Geometry check sheet. Reference: the model listing, model coordinates, mm. Face numbers are marked on the shaded views. Round coordinates to 2 decimals unless told otherwise and drop trailing zeros. Order: outer loops, then holes, each group sorted by start corner. A loop starts at its lowest first (then second) coordinate and runs counter-clockwise, first axis right, second up.
(1) Thickness scan on L1, parallel to Y at x = 0.95, z = 0; L2, parallel to Z at x = 2.2, y = -5.25. Record the ranges inside material, lowest first.
(2) Cross-section at D-D on y = -8. Enter the section's corners in (x, z).
(3) Cross-section at C-C on x = 1.4. Enter the section's corners in (y, z).
(4) Cross-section at A-A on y = 0. Enter the section's corners in (x, z).
(5) Cross-section at B-B on z = -4. Enter the section's corners in (x, y), and give its area (3 significant figures).
(6) Gauge pin test, flat ends, axial feed: P1, Ø10, axis at y = -7, z = -0.5, coming from the -X side; P2, Ø1.5, axis at x = 0.5, y = -1, coming from the +Z side. Record the tip position at first contact, or that the pin passes through.
(7) Draft check along X on the marked faces 1 and 2. Enter one of: pulls with the +X half, pulls with the -X half, needs draft (parallel to the pull), parting line crosses it, or undercut.
Autodesk Inventor part; units mm, degrees
ref_plane "Work Plane1" through (0, 0, 0) normal (0, -1, 0) x (1, 0, 0)
ref_plane "YZ Plane" through (0, 0, 0) normal (1, 0, 0) x (0, 1, 0)
ref_plane "XZ Plane" through (0, 0, 0) normal (0, 1, 0) x (-1, 0, 0)
sketch "草图1" plane through (0, 0, 0) normal (1, 0, 0) x (0, 1, 0)
  circle A0 centre (0, 0) radius 9.2
  circle A1 centre (0, 0) radius 6.1
  dimension "d0" = 12.2
  dimension "d1" = 18.4
extrude "轴承体" add sketch "草图1" along normal blind 3.1
sketch "草图2" plane through (0, 0, 0) normal (0, 0, 1) x (1, 0, 0)
  line L0 (0, -6.1) -> (0, 6.1)
  line L1 (3.1, 9.2) -> (3.1, -9.2)
  line L2 (-1.2, 0) -> (7.2, 0)
  line L3 (0, -0.62) -> (3.1, 0.3873)
  line L4 (0, 0.62) -> (3.1, 1.6273)
  dimension "d4" = 0.62
  dimension "d5" = 0.62
  dimension "d6" = 72
extrude "切口" cut sketch "草图2" along normal up to next contours L0 L2 L3 | L0 L4 L1 L3 L2
ref_plane "Work Plane1" through (0, 0, 0) normal (0, -1, 0) x (1, 0, 0)
equation "\"d0\" = SD1"
equation "\"d1\" = SD2"
equation "\"d2\" = SD"
equation "\"d4\" = 0.2 * SD"
equation "\"d5\" = 0.2 * SD"
equation "\"d6\" = FAWI"
equation "\"d7\" = SD"
equation "\"SD1\" = 12.2"
equation "\"SD2\" = 18.4"
equation "\"SD\" = 3.1"
equation "\"FAWI\" = 72deg"
equation "\"NND\" = 12"
properties part number "垫圈 GB 93-87 12" material "钢，软"
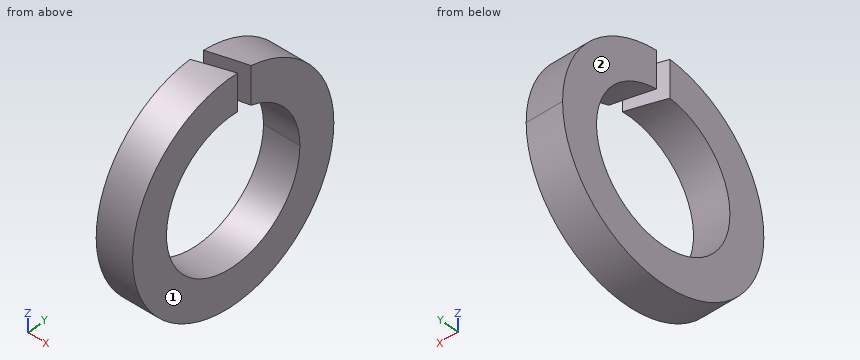
Found:
1. L1: y = -9.2 to -6.1, 6.1 to 9.2
1. L2: z = -7.55 to -3.11, 3.11 to 7.55
2. outline: (0, -4.54) - (3.1, -4.54) - (3.1, 4.54) - (0, 4.54) - close
3. outline: (-0.17, 6.1) - (-0.17, 9.2) arc R9.2 ccw (long way) to (1.07, 9.14) - (1.07, 6) arc R6.1 cw (long way) to start
4. outline: (0, -9.2) - (3.1, -9.2) - (3.1, -6.1) - (0, -6.1) - close; (1.91, 6.1) - (3.1, 6.1) - (3.1, 9.2) - (1.91, 9.2) - close
5. outline: (0, -8.28) - (3.1, -8.28) - (3.1, -4.61) - (0, -4.61) - close; (0, 4.61) - (3.1, 4.61) - (3.1, 8.28) - (0, 8.28) - close
5. area: 22.8 mm2
6. P1: stops at x = 0
6. P2: stops at z = 9.19
7. face 1: pulls with the +X half
7. face 2: pulls with the -X half
